Drawing for the job (mm, zero at the part's lowest x, y, z). A direction names the side the tool comes from. Coordinates: 2 decimals unless noted, no trailing zeros. Write each loop counter-clockwise with the first axis right and the second up, starting at its lowest first coordinate (ties: lowest second). Pieces come first, ordered by that corner, then holes. Notation, with made-up numbers: M 15.25,-6 L 43.25,-6 A31 cw 43.25,23 Z; hole C 53.25,-13.75 d1. An arc over 180 degrees is marked long. Use a Markdown table: item, result. Add a question column.
Q1. Pin check, flat tips, straight feed: pin 1 Ø3 at (y, z) = (2.5, 5.5) entering from -X; pin 2 Ø3 at (y, z) = (12.5, 36.5) entering from +X; pin 3 Ø5 at (x, y) = (6, 17.5) entering from -Z. Stop position of each tip, or through.
Q2. Slice it at D-D on y = 3.75. Write the cut outline in (x, z) (3 decimals), then the cut area to 3 significant figures.
Q3. Wall check: L1, parallel to Z at x = 22, y = 10.5 (3 decimals); L2, parallel to Z at x = 22, y = 17; L3, parallel to X at y = 20.75, z = 17. Give the ranges that are in metal, low to high. Write a range as from..to.
Q4. Tool access for the marked faces 4 and 5: list every direction of +Z, -Z, +X, -X, +Y, -Y with a clear straight run to the whole face (end or side of a thin tool).
Q5. Slice it at C-C on y = 22.25. Write the cut outline in (x, z).
Q6. Mould opens along X. For the marked faces 1, 2 and 3 say: released by +X, released by -X, zero draft, split by the parting line, or undercut.
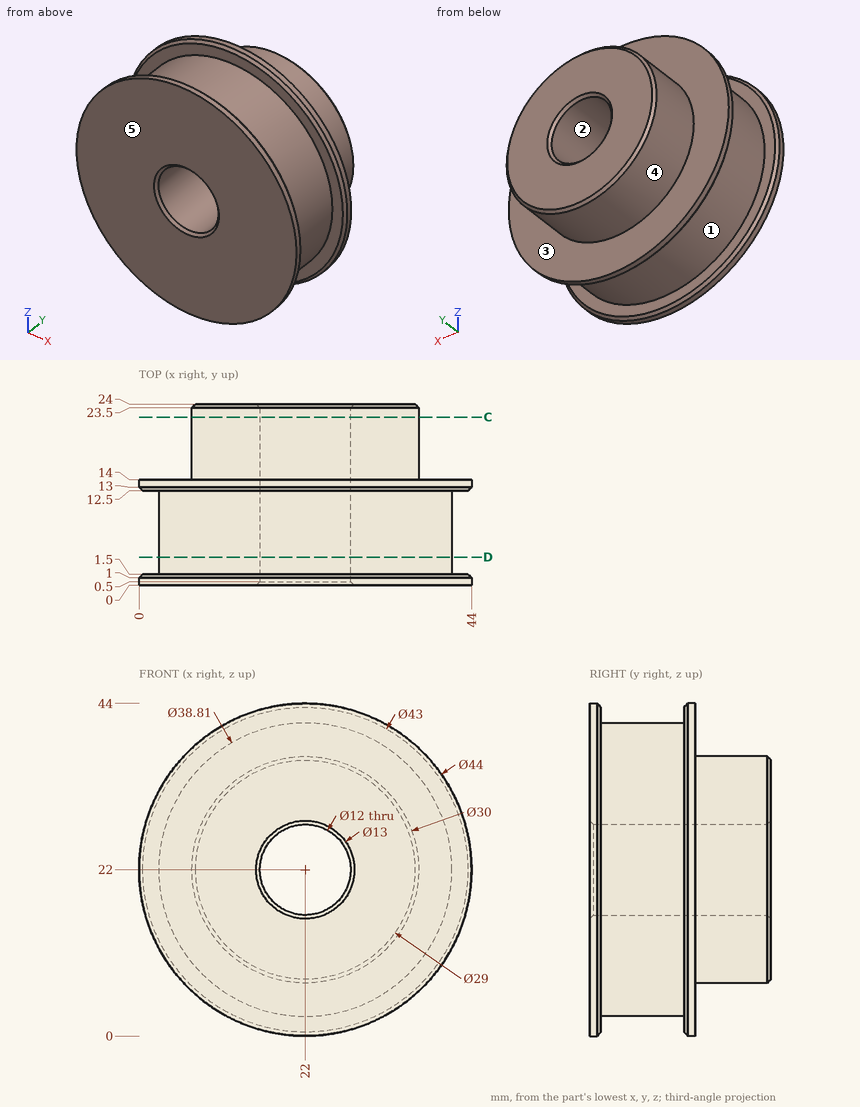
Recorded:
| question | item | result |
|---|---|---|
| 1 | pin 1 | x = 6.92 |
| 1 | pin 2 | x = 39.69 |
| 1 | pin 3 | z = 15.46 |
| 2 | outline | C 22,22 d38.81; hole C 22,22 d12 |
| 2 | area | 1,070 mm² |
| 3 | L1 | 2.595..16, 28..41.405 |
| 3 | L2 | 7..16, 28..37 |
| 3 | L3 | 7.86..18.68, 25.32..36.14 |
| 4 | face 4 | +Y |
| 4 | face 5 | +Z, -Z, +X, -X, -Y |
| 5 | outline | C 22,22 d30; hole C 22,22 d12 |
| 6 | face 1 | split by the parting line |
| 6 | face 2 | undercut |
| 6 | face 3 | zero draft |
